Geometry check sheet. Reference: the model listing, model coordinates, mm. A direction names the side the tool comes from. Coordinates: 2 decimals unless noted, no trailing zeros. Loops run counter-clockwise (first coordinate to the right, second up) from the corner with the lowest first, then second, coordinate; pieces in that order, holes last.
from build123d import *

# Parameters (mm, degrees)
SKETCH_1_R      = 1.75
EXTRUDE_1_DEPTH = 3


with BuildPart() as part:
    # 草圖1 → 填料-伸長1 (new body)
    with BuildSketch(Plane(origin=(0, 0, 0), x_dir=(1, 0, 0), z_dir=(0, 1, 0))):
        with BuildLine():
            Line((36.848566664, -25.260597764), (0, -80))
            ThreePointArc((0, -80), (14.411400344, -74.478032661), (25.446019232, -63.68832603))
            Line((25.446019232, -63.68832603), (47.47618504, -30.962002684))
            ThreePointArc((47.47618504, -30.962002684), (48.715425732, -28.156234166), (48.907790247, -25.095017029))
            Line((48.907790247, -25.095017029), (45.961176943, 0.681446592))
            ThreePointArc((45.961176943, 0.681446592), (43.994453683, 4.477090548), (40, 6))
            Line((40, 6), (0, 6))
            ThreePointArc((0, 6), (-6, 0), (0, -6))
            Line((0, -6), (34.646808717, -6))
            Line((34.646808717, -6), (36.848566664, -25.260597764))
        make_face()
        with Locations((40, 0)):
            Circle(SKETCH_1_R, mode=Mode.SUBTRACT)
        Circle(SKETCH_1_R, mode=Mode.SUBTRACT)
    extrude(amount=EXTRUDE_1_DEPTH)


solid = part.part
1) Material ranges on probe 1 along X at (y, z) = (1.65, 0); probe 2 along Z at (x, y) = (40, 1.8); probe 3 along Z at (x, y) = (11.5, 0.9), recorded low to high.
Data:
probe 1: x = -6 to -1.75, 1.75 to 38.25, 41.75 to 46.04
probe 2: z = -6 to -1.75, 1.75 to 42.07
probe 3: z = -6 to 6, 62.92 to 76.17
2) Mould release check, pull along Z, two halves, no side actions. Record for faces 3 (the cylindrical face through (1.617, 1.479, 0.67)), 4 (the flat face through (47.455, 1.479, 12.387)), 5 (the cylindrical face through (41.617, 1.479, 0.67)), 6 (the flat face through (36.31, 1.48, 47.55)): +Z half, -Z half, draft (parallel to the pull), parting line (faces both ways), or undercut.
Data:
face 3: undercut
face 4: -Z half
face 5: undercut
face 6: +Z half
3) Section check A-A on y = 1.1. Record the cut outline in (x, z).
Data:
outline: (0, -6) - (40, -6) arc R6 ccw to (45.96, -0.68) - (48.91, 25.1) arc R8.73 ccw to (47.48, 30.96) - (25.45, 63.69) arc R38.07 ccw to (0, 80) - (36.85, 25.26) - (34.65, 6) - (0, 6) arc R6 ccw to start; hole circle Ø3.5 at (0, 0); hole circle Ø3.5 at (40, 0)
4) Depth check by flat-ended pin: pin 1 (2 mm diameter, centred on x = 0, z = 0, fed in from +Y); pin 2 (0.9 mm diameter, centred on x = 25.5, y = 1.5, fed in from +Z). Enter the tip coordinate at first touch or a pass-through.
Data:
pin 1: passes through
pin 2: stops at z = 64.27
5) Section check B-B on x = 9. Record the cut outline in (y, z).
Data:
outline: (0, -6) - (3, -6) - (3, 6) - (0, 6) - close; (0, 66.63) - (3, 66.63) - (3, 77.36) - (0, 77.36) - close
6) Section check C-C on z = 23. Record the cut outline in (x, y), and give its area (3 significant figures).
Data:
outline: (36.59, 0) - (48.67, 0) - (48.67, 3) - (36.59, 3) - close
area: 36.2 mm2
7) Access from +Z, -Z, +X, -X, +Y, -Y to the whole of each face (thin tool, end or side, straight path). Record for faces 1 (the flat face through (35.732, 1.479, 15.495)), 2 (the cylindrical face through (14.228, 1.479, 74.595)).
Data:
face 1: -X, +Y, -Y
face 2: +Z, +X, +Y, -Y
8) Section check D-D on x = -3. Record the cut outline in (y, z), and give its area (3 significant figures).
Data:
outline: (0, -5.2) - (3, -5.2) - (3, 5.2) - (0, 5.2) - close
area: 31.2 mm2
